```python
from build123d import *

# Parameters (mm, degrees)
F1_DEPTH = 10
F2_R     = 2.25
F3_DEPTH = 25
F4_R     = 2.25
F5_DEPTH = 3


with BuildPart() as f1:
    # F0 (on Top) → F1 (new body, symmetric)
    with BuildSketch(Plane.XY):
        with BuildLine():
            Line((-35, 7), (-35, 0))
            Line((-35, 0), (-14.142136, 0))
            ThreePointArc((-14.142136, 0), (0, 10), (14.142136, 0))
            Line((14.142136, 0), (35, 0))
            Line((35, 0), (35, 7))
            Line((35, 7), (18.439089, 7))
            ThreePointArc((18.439089, 7), (0, 17), (-18.439089, 7))
            Line((-18.439089, 7), (-35, 7))
        make_face()
    extrude(amount=F1_DEPTH, both=True)

    # F2 (on face) → F3 (cut)
    with BuildSketch(Plane(origin=(0, 7, 0), x_dir=(-1, 0, 0), z_dir=(0, 1, 0))):
        with Locations((-26.719544, 0)):
            Circle(F2_R)
        with Locations((26.719544, 0)):
            Circle(F2_R)
    extrude(amount=-F3_DEPTH, mode=Mode.SUBTRACT)

    # F4 (on face) → F5 (cut)
    with BuildSketch(Plane(origin=(0, 7, 0), x_dir=(-1, 0, 0), z_dir=(0, 1, 0))):
        Polygon((-28.74027, 3.5), (-30.760996, 0), (-28.74027, -3.5), (-24.698819, -3.5), (-22.678093, 0), (-24.698819, 3.5), align=None)
        with Locations((-26.719544, 0)):
            Circle(F4_R, mode=Mode.SUBTRACT)
        Polygon((28.74027, -3.5), (30.760996, 0), (28.74027, 3.5), (24.698819, 3.5), (22.678093, 0), (24.698819, -3.5), align=None)
    extrude(amount=-F5_DEPTH, mode=Mode.SUBTRACT)


solid = f1.part
```
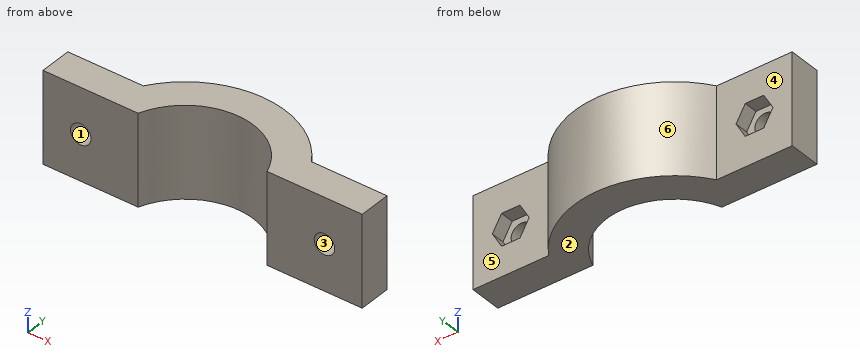
The listing builds one solid part. Answer for the finished solid, in the listing's coordinates (mm). Face numbers are marked on the shaded views. A direction names the side the tool comes from. Give positions to 0.01 mm unless a question says otherwise; leave off trailing zeros. Order: outer loops, then holes, each group sorted by start corner. A loop starts at its lowest first (then second) coordinate and runs counter-clockwise, first axis right, second up. Notation, with made-up numbers: (27.5, -9.5) - (44.5, -9.5) arc R22 cw to (44.5, 1.5) - close; hole circle Ø1 at (89, -27). An arc over 180 degrees is marked (long way). Answer in a Markdown table with one row per item. Add a question column.
Q1. Which of the six approach directions +Z, -Z, +X, -X, +Y, -Y give full straight-line access (tool end or side, diameter ignored) to the marked faces 5 and 6?
Q2. The part is cut by section B-B (z = -7.25). Determine the outline of the cut face in (x, y).
Q3. For a pull along Z with two mould halves and no side action, classify the marked faces 1, 2, 3 and 4 as released by +Z, released by -Z, zero draft, split by the parting line, or undercut.
Q4. The part is cut by section C-C (x = -25.5). Determine the outline of the cut face in (y, z), then the cut area to 3 significant figures.
Q5. The part is cut by section D-D (y = 8). Determine the outline of the cut face in (x, z), then the cut area to 3 significant figures.
Q6. Find the intervals of material crossed by line 1 along X through (y, z) = (4.5, 3.25); line 2 along Z through (x, y) = (26.5, 2); line 3 along X through (y, z) = (5, 2.5), in increasing order. Write a range as [from, to].
Q7. Given P1, Ø1, axis at x = 11.5, z = 7, coming from the +Y side; P2, Ø2, axis at x = 12.5, y = 13.5, coming from the +Z side; P3, Ø7.5, axis at x = 28.5, z = -1.5, coming from the +Y side; P4, Ø1.5, axis at y = 10.5, z = -1.5, coming from the -X side, each flat-ended and moving along its own axis, determine where each tip first touches the part or whether it passes through.
Q8. The part is cut by section A-A (y = 1.5). Determine the outline of the cut face in (x, z), then the cut area to 3 significant figures.
Determined:
| question | item | result |
|---|---|---|
| 1 | face 5 | +Z, -Z, +X, +Y |
| 1 | face 6 | +Z, -Z, +Y |
| 2 | outline | (-35, 0) - (-14.14, 0) arc R15 cw to (14.14, 0) - (35, 0) - (35, 7) - (18.44, 7) arc R22 ccw to (-18.44, 7) - (-35, 7) - close |
| 3 | face 1 | undercut |
| 3 | face 2 | released by -Z |
| 3 | face 3 | undercut |
| 3 | face 4 | zero draft |
| 4 | outline | (0, -10) - (7, -10) - (7, -3.5) - (4, -3.5) - (4, -1.89) - (0, -1.89) - close; (0, 1.89) - (4, 1.89) - (4, 3.5) - (7, 3.5) - (7, 10) - (0, 10) - close |
| 4 | area | 104 mm² |
| 5 | outline | (-17.75, -10) - (-7.48, -10) - (-7.48, 10) - (-17.75, 10) - close; (7.48, -10) - (17.75, -10) - (17.75, 10) - (7.48, 10) - close |
| 5 | area | 411 mm² |
| 6 | line 1 | x = [-35, -28.88], [-24.55, -11.61], [11.61, 24.55], [28.88, 35] |
| 6 | line 2 | z = [-10, -2.24], [2.24, 10] |
| 6 | line 3 | x = [-35, -29.32], [-24.12, -11.18], [11.18, 24.12], [29.32, 35] |
| 7 | P1 | stops at y = 14.05 |
| 7 | P2 | stops at z = 10 |
| 7 | P3 | stops at y = 7 |
| 7 | P4 | stops at x = -16.32 |
| 8 | outline | (-35, -10) - (-13.52, -10) - (-13.52, 10) - (-35, 10) - close; (13.52, -10) - (35, -10) - (35, 10) - (13.52, 10) - close; hole circle Ø4.5 at (-26.72, 0); hole circle Ø4.5 at (26.72, 0) |
| 8 | area | 827 mm² |
